Autodesk Inventor part; units mm, degrees
ref_plane "Plano inicial" through (0, 0, -25) normal (0, 0, 1) x (1, 0, 0)
ref_plane "Plano final" through (0, 0, 2340) normal (0, 0, 1) x (1, 0, 0)
ref_plane "Plano de trabajo4" through (0, -21, -25) normal (0, 0, -1) x (-1, 0, 0)
ref_plane "Plano inicial" through (0, 0, -25) normal (0, 0, 1) x (1, 0, 0)
ref_plane "Plano final" through (0, 0, 2340) normal (0, 0, 1) x (1, 0, 0)
sketch "Boceto" plane through (0, 0, 0) normal (0, 0, 1) x (1, 0, 0)
  line L0 (-35, -29) -> (-35, 29)
  line L1 (-29, 35) -> (29, 35)
  line L2 (35, 29) -> (35, -29)
  line L3 (29, -35) -> (-29, -35)
  arc A0 (-35, -29) -> (-29, -35) centre (-29, -29) ccw
  arc A1 (35, 29) -> (29, 35) centre (29, 29) ccw
  arc A2 (-29, 35) -> (-35, 29) centre (-29, 29) ccw
  arc A3 (29, -35) -> (35, -29) centre (29, -29) ccw
  arc A4 (-29, 32) -> (-32, 29) centre (-29, 29) ccw
  line L4 (-29, 32) -> (29, 32)
  arc A5 (32, 29) -> (29, 32) centre (29, 29) ccw
  line L5 (32, 29) -> (32, -29)
  arc A6 (29, -32) -> (32, -29) centre (29, -29) ccw
  line L6 (29, -32) -> (-29, -32)
  arc A7 (-32, -29) -> (-29, -32) centre (-29, -29) ccw
  line L7 (-32, -29) -> (-32, 29)
  line L8 (0, 50.7397) -> (0, -50.7397) construction
  line L9 (-50.7397, 0) -> (50.7397, 0) construction
  dimension "d7" = 6
  dimension "d9" = 70
  dimension "d11" = 70
  dimension "d12" = 3
  dimension "d15" = 35
  dimension "d16" = 35
extrude "Cuerpo" add sketch "Boceto" along normal up to surface (2365 mm away) from surface at -25
sketch "Sketch3" plane through (0, 0, 0) normal (0, 0, 1) x (1, 0, 0)
  line L0 (0, 0) -> (10, 0)
ref_plane "Work Plane3" through (0, 0, 0) normal (0, -1, 0) x (1, 0, 0)
sketch "Sketch4" plane through (0, 0, 0) normal (0, -1, 0) x (1, 0, 0)
  line L0 (-2, -25) -> (12, -25)
  line L1 (-2, 2340) -> (12, 2340)
  dimension "d18" = 2365
ref_plane "Plano de trabajo4" through (0, -21, -25) normal (0, 0, -1) x (-1, 0, 0)
split "Dividir1" plane through (0, -21, -25) removes the side toward (0, 0, -1)
ref_plane "Plano de trabajo5" through (-500, -21, 2340) normal (0, 0, 1) x (1, 0, 0)
split "Dividir2" plane through (-500, -21, 2340) removes the side toward (0, 0, 1)
equation "\"d7\" = G_IR"
equation "\"d9\" = G_W"
equation "\"d11\" = G_H"
equation "\"d12\" = G_T"
equation "\"d15\" = 0.5 * d9"
equation "\"d16\" = 0.5 * d11"
equation "\"d3\" = G_L"
equation "\"G_W\" = 70"
equation "\"G_H\" = 70"
equation "\"G_T\" = 3"
equation "\"G_IR\" = 6"
equation "\"G_L\" = d18"
equation "\"G_OFFSET_START\" = 25"
equation "\"G_OFFSET_END\" = 25"
equation "\"d13\" = -G_OFFSET_START"
equation "\"B_L\" = 2315"
properties part number "ISO 10799-2 - 70x70x3 - 2365" material "Galvanizado catalogo 2"
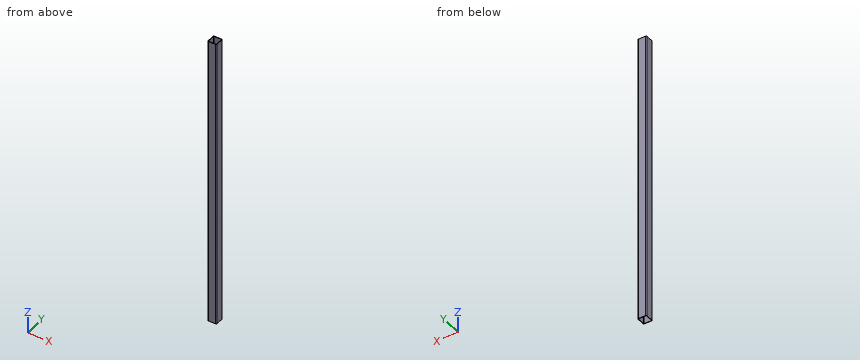
Build history of the part. All positions in model axes, mm. Round coordinates to 2 decimals unless told otherwise and drop trailing zeros. Write each loop counter-clockwise with the first axis right and the second up, starting at its lowest first coordinate (ties: lowest second). Pieces come first, ordered by that corner, then holes. Notation, with made-up numbers: (60.25, 71) - (119.25, 71) arc R15 cw to (119.25, 87) - close; hole circle Ø7 at (60, 77). An arc over 180 degrees is marked (long way). Answer as CSV lines item,"result".
Q1. Cut at A-A (y = -8). Write the cut outline in (x, z), and give its area (3 significant figures).
Report:
outline,"(-35, -25) - (-32, -25) - (-32, 2340) - (-35, 2340) - close; (32, -25) - (35, -25) - (35, 2340) - (32, 2340) - close"
area,"14,200 mm^2"
Q2. Drill centre lines: probe 1 along X at (y, z) = (8, 451.5); probe 2 along Y at (x, z) = (-31, 1665). Where is each one in solid material? Low to high. Write a range as [from, to].
Report:
probe 1,"x = [-35, -32], [32, 35]"
probe 2,"y = [-34.66, -31.24], [31.24, 34.66]"
Q3. Cut at C-C (z = 193). Write the cut outline in (x, y), and give its area (3 significant figures).
Report:
outline,"(-35, -29) arc R6 ccw to (-29, -35) - (29, -35) arc R6 ccw to (35, -29) - (35, 29) arc R6 ccw to (29, 35) - (-29, 35) arc R6 ccw to (-35, 29) - close; hole (-32, -29) arc R3 ccw to (-29, -32) - (29, -32) arc R3 ccw to (32, -29) - (32, 29) arc R3 ccw to (29, 32) - (-29, 32) arc R3 ccw to (-32, 29) - close"
area,"781 mm^2"
